Input: part model. Units: mm. Frame: model coordinates. A direction names the side the tool comes from. Round coordinates to 2 decimals unless told otherwise and drop trailing zeros. Loops run counter-clockwise (first coordinate to the right, second up) from the corner with the lowest first, then second, coordinate; pieces in that order, holes last. Notation, with made-up numbers: (33, 88.5) -> (87, 88.5) arc R35 cw to (87, 120.5) -> close; hole circle Ø6 at (88, 18.25). An arc over 180 degrees is marked (long way). Answer as a JSON object with one key per item and string values.
Autodesk Inventor part; units mm, degrees
ref_plane "YZ Plane" through (0, 0, 0) normal (1, 0, 0) x (0, 1, 0)
ref_plane "XZ Plane" through (0, 0, 0) normal (0, 1, 0) x (-1, 0, 0)
ref_plane "XY Plane" through (0, 0, 0) normal (0, 0, 1) x (1, 0, 0)
sketch "Sketch2" plane through (0, 0, 0) normal (0, 0, 1) x (1, 0, 0)
  line L0 (0, 0) -> (200, 0)
  line L1 (200, 0) -> (200, 150)
  line L2 (200, 150) -> (0, 150)
  line L3 (0, 150) -> (0, 0)
  circle A0 centre (100, 75) radius 15
  dimension "d4" = 150
  dimension "d5" = 200
  dimension "d6" = 75
  dimension "d7" = 100
  dimension "d8" = 30
extrude "Extrusion2" add sketch "Sketch2" against normal blind 10
sketch "Sketch6" plane through (0, 0, -10) normal (0, 0, -1) x (-1, 0, 0)
  line L0 (0, 150) -> (-200, 150)
  line L1 (0, 0) -> (0, 150)
  point P0 (-30, 75)
  point P1 (-170, 75)
  dimension "d28" = 75
  dimension "d29" = 75
  dimension "d30" = 140
  dimension "d31" = 30
hole "Hole2" at (30, 75, -10) at (170, 75, -10) direction (0, 0, 1) diameter 6.647 end through all counterbore diameter 14 counterbore depth 5
sketch "Sketch7" plane through (0, 0, 0) normal (0, 0, 1) x (1, 0, 0)
  circle A0 centre (83.75, 91.25) radius 3
  circle A1 centre (116.25, 91.25) radius 3
  circle A2 centre (83.75, 58.75) radius 3
  circle A3 centre (116.25, 58.75) radius 3
  circle A4 centre (100, 75) radius 15
  point P0 (0, 0)
  dimension "d39" = 16.25
  dimension "d40" = 16.25
  dimension "d41" = 16.25
  dimension "d42" = 16.25
  dimension "d43" = 16.25
  dimension "d44" = 16.25
  dimension "d45" = 16.25
  dimension "d46" = 16.25
  dimension "d47" = 6
extrude "Extrusion5" cut sketch "Sketch7" against normal blind 15 contours A0 | A1 | A2 | A3
sketch "Sketch8" plane through (0, 0, 0) normal (0, 0, 1) x (1, 0, 0)
  circle A0 centre (83.75, 91.25) radius 3
  circle A1 centre (116.25, 91.25) radius 3
  circle A2 centre (83.75, 58.75) radius 3
  circle A3 centre (116.25, 58.75) radius 3
  circle A4 centre (83.75, 91.25) radius 5.25
  circle A5 centre (116.25, 91.25) radius 5.25
  circle A6 centre (83.75, 58.75) radius 5.25
  circle A7 centre (116.25, 58.75) radius 5.25
  point P0 (0, 0)
  dimension "d50" = 10.5
  dimension "d51" = 10.5
  dimension "d52" = 10.5
  dimension "d53" = 10.5
extrude "Extrusion6" cut sketch "Sketch8" against normal blind 6 contours A0 | A2 | A3 | A4 | A5 | A6 | A7
equation "\"d40\" = d39"
equation "\"d41\" = d39"
equation "\"d42\" = d39"
equation "\"d43\" = d39"
equation "\"d44\" = d39"
equation "\"d45\" = d39"
equation "\"d46\" = d39"
equation "\"d50\" = d52"
equation "\"d51\" = d52"
equation "\"d53\" = d52"
properties part number "Soporte Piston"
1) Section B-B, the plane x = 100. Output: boundary loops of the cut face in (y, z), plus the area to 3 significant figures.
Output:
{"outline": "(0, -10) -> (60, -10) -> (60, 0) -> (0, 0) -> close; (90, -10) -> (150, -10) -> (150, 0) -> (90, 0) -> close", "area": "1,200 mm^2"}
2) Section A-A, the plane z = -3.5. Output: boundary loops of the cut face in (x, y), plus the area to 3 significant figures.
Output:
{"outline": "(0, 0) -> (200, 0) -> (200, 150) -> (0, 150) -> close; hole circle Ø6.65 at (30, 75); hole circle Ø10.5 at (83.75, 58.75); hole circle Ø10.5 at (83.75, 91.25); hole circle Ø30 at (100, 75); hole circle Ø10.5 at (116.25, 58.75); hole circle Ø10.5 at (116.25, 91.25); hole circle Ø6.65 at (170, 75)", "area": "28,900 mm^2"}
3) Ray query, probe 1 along Y at (x, z) = (83.75, -1.4); probe 2 along Y at (x, z) = (83.75, -8.9); probe 3 along Y at (x, z) = (30, -8.45). Return the intervals inside material, ascending.
Output:
{"probe 1": "y = 0 to 53.5, 64 to 86, 96.5 to 150", "probe 2": "y = 0 to 55.75, 61.75 to 88.25, 94.25 to 150", "probe 3": "y = 0 to 68, 82 to 150"}
4) Draft query along X for faces 4 (the face through (119, 89, -6)), 5 (the face through (0, 76, -5)), 6 (the face through (101, 150, -5)). Return one class per face: +X half, -X half, draft (parallel to the pull), parting line (faces both ways), or undercut.
Output:
{"face 4": "undercut", "face 5": "-X half", "face 6": "draft"}
5) Contact query for flat-ended pins moving along their axis: P1, Ø5, axis at x = 84.5, y = 59.5, coming from the +Z side; P2, Ø11, axis at x = 29.5, y = 78, coming from the -Z side; P3, Ø11, axis at x = 30, y = 75, coming from the -Z side; P4, Ø3.5, axis at x = 116.25, y = 58.75, coming from the -Z side. Output: stop coordinate, or through.
Output:
{"P1": "stops at z = -6", "P2": "stops at z = -10", "P3": "stops at z = -5", "P4": "passes through"}
6) Reachability of faces 1 (the face through (117.634, 88.588, -7.972)), 2 (the face through (119, 56, -6)), 3 (the face through (173, 73, -5)) from +Z, -Z, +X, -X, +Y, -Y: full face, straight path, thin tool, end or side. Return the list, or none.
Output:
{"face 1": "+Z, -Z", "face 2": "+Z", "face 3": "-Z"}
